Check sheet for the modelled part. Datum: model origin and axes. Units: mm. Face numbers are marked on the shaded views. A direction names the side the tool comes from. Round coordinates to 2 decimals unless told otherwise and drop trailing zeros. Order: outer loops, then holes, each group sorted by start corner. A loop starts at its lowest first (then second) coordinate and runs counter-clockwise, first axis right, second up. Notation, with made-up numbers: (-38, -35) -> (-26, -35) arc R17 cw to (-26, -30) -> close; hole circle Ø8 at (56.5, 68). An arc over 180 degrees is marked (long way). Answer in a Markdown table with one row per item. Add a question column.
1. Material ranges on L1, parallel to X at y = 4, z = 38; L2, parallel to Z at x = -25.4, y = 4 (3 decimals); L3, parallel to Y at x = 5, z = 0, recorded low to high. Write a range as from..to.
2. Draft check along Y on the marked faces 4, 5 and 6. Enter one of: +Y half, -Y half, draft (parallel to the pull), parting line (faces both ways), or undercut.
3. Sectioned sample at D-D, the plane y = 105. Record the boundary of the cut face in (x, z).
4. Sectioned sample at B-B, the plane x = -25.4. Record the boundary of the cut face in (y, z) (3 decimals), then the cut area to 3 significant figures.
5. Access from +Z, -Z, +X, -X, +Y, -Y to the whole of each face (thin tool, end or side, straight path). Record for the marked faces 1, 2 and 3.
6. Depth check by flat-ended pin: P1, Ø4, axis at y = 69, z = -12, coming from the -X side; P2, Ø3, axis at x = 25.4, z = 38.1, coming from the +Y side; P3, Ø9, axis at x = -27.5, z = -6, coming from the +Y side; P4, Ø6, axis at x = 25.4, z = -38.1, coming from the -Y side. Enter the tip coordinate at first touch or a pass-through.
7. Sectioned sample at C-C, the plane z = -38.1. Record the boundary of the cut face in (x, y) (3 decimals).
8. Sectioned sample at A-A, the plane z = 0. Record the boundary of the cut face in (x, y), then the cut area to 3 significant figures.
```python
from build123d import *

# Parameters (mm, degrees)
SKETCH2_W           = 80
SKETCH2_H           = 100
BOSS_EXTRUDE1_DEPTH = 10
SKETCH3_W           = 20
SKETCH3_H           = 100
BOSS_EXTRUDE2_DEPTH = 120
SKETCH5_R           = 2.555
CUT_EXTRUDE2_DEPTH  = 55
SKETCH4_R           = 16.25
CUT_EXTRUDE4_DEPTH  = 45


with BuildPart() as part:
    # Sketch2 → Boss-Extrude1 (new body)
    with BuildSketch(Plane(origin=(0, 0, 0), x_dir=(1, 0, 0), z_dir=(0, 1, 0))):
        Rectangle(SKETCH2_W, SKETCH2_H)
    extrude(amount=BOSS_EXTRUDE1_DEPTH)

    # Sketch3 → Boss-Extrude2 (add)
    with BuildSketch(Plane(origin=(0, 10, 0), x_dir=(1, 0, 0), z_dir=(0, 1, 0))):
        Rectangle(SKETCH3_W, SKETCH3_H)
    extrude(amount=BOSS_EXTRUDE2_DEPTH)

    # Sketch5 → Cut-Extrude2 (cut)
    with BuildSketch(Plane.XZ):
        with Locations((-25.4, -38.1)):
            Circle(SKETCH5_R)
        with Locations((25.4, -38.1)):
            Circle(SKETCH5_R)
        with Locations((-25.4, 38.1)):
            Circle(SKETCH5_R)
        with Locations((25.4, 38.1)):
            Circle(SKETCH5_R)
    extrude(amount=-CUT_EXTRUDE2_DEPTH, mode=Mode.SUBTRACT)

    # Sketch4 → Cut-Extrude4 (cut)
    with BuildSketch(Plane.ZY.offset(10)):
        with Locations((0, 93.587135628)):
            Circle(SKETCH4_R)
    extrude(amount=-CUT_EXTRUDE4_DEPTH, mode=Mode.SUBTRACT)


solid = part.part
```
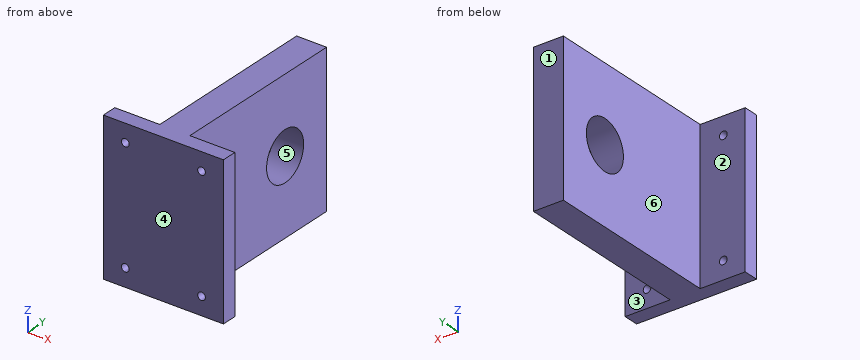
Answer key:
| question | item | result |
|---|---|---|
| 1 | L1 | x = -40..-27.95, -22.85..22.85, 27.95..40 |
| 1 | L2 | z = -50..-40.655, -35.545..35.545, 40.655..50 |
| 1 | L3 | y = 0..77.34, 109.84..130 |
| 2 | face 4 | -Y half |
| 2 | face 5 | undercut |
| 2 | face 6 | draft |
| 3 | outline | (-10, -50) -> (10, -50) -> (10, -11.57) -> (-10, -11.57) -> close; (-10, 11.57) -> (10, 11.57) -> (10, 50) -> (-10, 50) -> close |
| 4 | outline | (0, -50) -> (10, -50) -> (10, -40.655) -> (0, -40.655) -> close; (0, -35.545) -> (10, -35.545) -> (10, 35.545) -> (0, 35.545) -> close; (0, 40.655) -> (10, 40.655) -> (10, 50) -> (0, 50) -> close |
| 4 | area | 898 mm² |
| 5 | face 1 | +Z, -Z, +X, -X, +Y |
| 5 | face 2 | +Z, -Z, -X, +Y |
| 5 | face 3 | +Z, -Z, +X, +Y |
| 6 | P1 | stops at x = -10 |
| 6 | P2 | passes through |
| 6 | P3 | stops at y = 10 |
| 6 | P4 | stops at y = 0 |
| 7 | outline | (-40, 0) -> (-27.955, 0) -> (-27.955, 10) -> (-40, 10) -> close; (-22.845, 0) -> (22.845, 0) -> (22.845, 10) -> (10, 10) -> (10, 130) -> (-10, 130) -> (-10, 10) -> (-22.845, 10) -> close; (27.955, 0) -> (40, 0) -> (40, 10) -> (27.955, 10) -> close |
| 8 | outline | (-40, 0) -> (40, 0) -> (40, 10) -> (10, 10) -> (10, 77.34) -> (-10, 77.34) -> (-10, 10) -> (-40, 10) -> close; (-10, 109.84) -> (10, 109.84) -> (10, 130) -> (-10, 130) -> close |
| 8 | area | 2,550 mm² |
